For this review, take the finished solid that the model builds, in its own axes (mm). A direction names the side the tool comes from. Coordinates: 2 decimals unless noted, no trailing zeros. Order: outer loops, then holes, each group sorted by start corner. A loop starts at its lowest first (then second) coordinate and runs counter-clockwise, first axis right, second up.
from build123d import *

# Parameters (mm, degrees)
SKETCH3_R           = 3
BOSS_EXTRUDE1_DEPTH = 21
CUT_EXTRUDE1_DEPTH  = 5
SKETCH6_R           = 1.6
CUT_EXTRUDE2_DEPTH  = 10


with BuildPart() as part:
    # Sketch1 → Revolve1 (revolve)
    with BuildSketch(Plane(origin=(0, 0, 0), x_dir=(1, 0, 0), z_dir=(0, 1, 0))):
        with BuildLine():
            Line((0, 2), (0, -2))
            Line((0, -2), (5.656854249, -2))
            ThreePointArc((5.656854249, -2), (6, 0), (5.656854249, 2))
            Line((5.656854249, 2), (0, 2))
        make_face()
    revolve(axis=Axis((0, 0, -2), (0, 0, 1)))

    # Sketch3 → Boss-Extrude1 (add)
    with BuildSketch(Plane(origin=(0, 0, 0), x_dir=(1, 0, 0), z_dir=(0, 1, 0))):
        with Locations(Location((0, 0, 0), (0, 0, 270))):
            Circle(SKETCH3_R)
    extrude(amount=-BOSS_EXTRUDE1_DEPTH)

    # Sketch4 → Cut-Revolve2 (revolve, cut)
    with BuildSketch(Plane(origin=(0, 0, 0), x_dir=(1, 0, 0), z_dir=(0, 1, 0))):
        with BuildLine():
            Line((0, 3.9), (0, -3.9))
            ThreePointArc((0, -3.9), (3.9, 0), (0, 3.9))
        make_face()
    revolve(axis=Axis((0, 0, -3.9), (0, 0, 1)), mode=Mode.SUBTRACT)

    # Sketch5 → Cut-Extrude1 (cut, symmetric)
    with BuildSketch(Plane(origin=(0, 0, 0), x_dir=(0, 0, -1), z_dir=(1, 0, 0))):
        Polygon((2, -5.196152423), (3, -5.491987159), (3, -2.491987159), (2, -2.491987159), align=None)
        Polygon((-2, -2.491987159), (-3, -2.491987159), (-3, -5.491987159), (-2, -5.196152423), align=None)
    extrude(amount=CUT_EXTRUDE1_DEPTH, both=True, mode=Mode.SUBTRACT)

    # Sketch6 → Cut-Extrude2 (cut)
    with BuildSketch(Plane.XZ.offset(21)):
        with Locations(Location((0, 0, 0), (0, 0, 270))):
            Circle(SKETCH6_R)
    extrude(amount=-CUT_EXTRUDE2_DEPTH, mode=Mode.SUBTRACT)


solid = part.part
1. Take a section at A-A, the plane z = 0. Give the boundary of the cut face in (x, y), plus the area to 3 significant figures.
Answer below:
outline: (-3, -21) - (-1.6, -21) - (-1.6, -11) - (1.6, -11) - (1.6, -21) - (3, -21) - (3, -5.2) arc R6 ccw (long way) to (-3, -5.2) - close; hole circle Ø7.8 at (0, 0)
area: 125 mm2
2. Take a section at C-C, the plane y = -0.5. Give the boundary of the cut face in (x, z), plus the area to 3 significant figures.
Answer below:
outline: (-5.63, -2) - (-3.31, -2) arc R3.87 cw to (-3.31, 2) - (-5.63, 2) arc R5.98 ccw to start; (3.31, -2) - (5.63, -2) arc R5.98 ccw to (5.63, 2) - (3.31, 2) arc R3.87 cw to start
area: 17.4 mm2
3. The part is to be moulded in two halves that separate along Z. For faces 1 (the face through (0, -11, 0)), 2 (the face through (0.031, -5.313, 2.396)), 3 (the face through (-0.03, -5.31, -2.38)), 4 (the face through (-0.97, -16.07, 1.27)), say which applies: +Z half, -Z half, draft (parallel to the pull), parting line (faces both ways), or undercut.
Answer below:
face 1: undercut
face 2: +Z half
face 3: -Z half
face 4: undercut
4. To check wall thickness, follow L1, parallel to X at y = -16, z = 0; L2, parallel to Z at x = -2, y = -18.5; L3, parallel to Y at x = -2.75, z = -1. State the ranges of each line that lie inside material, in increasing order.
Answer below:
L1: x = -3 to -1.6, 1.6 to 3
L2: z = -2.24 to 2.24
L3: y = -21 to -2.58, 2.58 to 5.24
5. Clearance check with flat-ended pins moving along their axes: pin 1 Ø3 at (x, z) = (3.5, -1.5) entering from +Y; pin 2 Ø1.9 at (x, z) = (0, 0) entering from -Y; pin 3 Ø5 at (x, y) = (-2.5, 0.5) entering from +Z. State where each tip first meets the part, or that it passes through.
Answer below:
pin 1: stops at y = 5.54
pin 2: stops at y = -11
pin 3: stops at z = 2
6. Take a section at D-D, the plane y = -17.75. Give the boundary of the cut face in (x, z).
Answer below:
outline: circle Ø6 at (0, 0); hole circle Ø3.2 at (0, 0)
7. Machinability: for faces 5 (the face through (2, 3, -2)), 6 (the face through (-2, 3, 2)), 7 (the face through (0.9, -12.99, 2.86)), 8 (the face through (-1.3, -21, 1.3)), which of the approach directions +Z, -Z, +X, -X, +Y, -Y give a long, thin tool a straight path to every point of the face, cutting with its end or side? Answer none if there is none.
Answer below:
face 5: -Z, +X, -X, +Y
face 6: +Z, +X, -X, +Y
face 7: -Y
face 8: +Z, -Z, +X, -X, -Y
8. Take a section at B-B, the plane x = 0. Give the boundary of the cut face in (y, z).
Answer below:
outline: (-21, -3) - (-5.49, -3) - (-5.2, -2) - (-3.35, -2) arc R3.9 cw to (-3.35, 2) - (-5.2, 2) - (-5.49, 3) - (-21, 3) - (-21, 1.6) - (-11, 1.6) - (-11, -1.6) - (-21, -1.6) - close; (3.35, -2) - (5.66, -2) arc R6 ccw to (5.66, 2) - (3.35, 2) arc R3.9 cw to start
